Autodesk Inventor part; units mm, degrees
ref_plane "YZ Plane" through (0, 0, 0) normal (1, 0, 0) x (0, 1, 0)
ref_plane "XZ Plane" through (0, 0, 0) normal (0, 1, 0) x (-1, 0, 0)
ref_plane "XY Plane" through (0, 0, 0) normal (0, 0, 1) x (1, 0, 0)
sketch "Sketch1" plane through (0, 0, 0) normal (0, 0, 1) x (1, 0, 0)
  line L0 (0, 0) -> (125, 0)
  line L1 (125, 0) -> (125, 64)
  line L2 (125, 64) -> (0, 64)
  line L3 (0, 64) -> (0, 0)
  line L4 (0, 64) -> (14.15, 64) construction
  line L5 (14.15, 64) -> (14.15, 57.7) construction
  line L6 (14.15, 57.7) -> (110.85, 57.7)
  line L7 (110.85, 57.7) -> (110.85, 6.3)
  line L8 (110.85, 6.3) -> (14.15, 6.3)
  line L9 (14.15, 6.3) -> (14.15, 57.7)
  line L10 (0, 64) -> (0, 57.85) construction
  line L11 (0, 57.85) -> (6, 57.85) construction
  line L12 (6, 57.85) -> (6, 32.1) construction
  line L13 (6, 32.1) -> (6, 6.35) construction
  line L14 (6, 6.35) -> (119, 6.35) construction
  line L15 (119, 6.35) -> (119, 32.1) construction
  line L16 (119, 32.1) -> (119, 57.85) construction
  circle A0 centre (6, 57.85) radius 1.5
  circle A1 centre (6, 32.1) radius 1.5
  circle A2 centre (6, 6.35) radius 1.5
  circle A3 centre (119, 6.35) radius 1.5
  circle A4 centre (119, 57.85) radius 1.5
  circle A5 centre (119, 32.1) radius 1.5
  dimension "d0" = 125
  dimension "d1" = 64
  dimension "d2" = 14.15
  dimension "d3" = 6.3
  dimension "d4" = 96.7
  dimension "d5" = 51.4
  dimension "d6" = 6.15
  dimension "d7" = 6
  dimension "d8" = 25.75
  dimension "d9" = 25.75
  dimension "d10" = 113
  dimension "d11" = 3
  dimension "d12" = 3
  dimension "d13" = 3
  dimension "d14" = 3
  dimension "d16" = 3
  dimension "d18" = 3
extrude "Plate2" add sketch "Sketch1" along normal blind 0.5
sketch "Sketch2" plane through (0, 0, 0.5) normal (0, 0, 1) x (1, 0, 0)
  line L0 (0, 0) -> (125, 0)
  line L1 (125, 0) -> (125, -1)
  line L2 (125, -1) -> (0, -1)
  line L3 (0, -1) -> (0, 0)
  dimension "d20" = 125
  dimension "d21" = 1
sheet face with bend "Face3" sketch "Sketch2" thickness 0.5 toward (0, 0, -1) bend radius 0.5
bend "Bend1"
sketch "Sketch4" plane through (0, -1, 0.5) normal (0, -1, 0) x (1, 0, 0)
  line L0 (0, -0.5) -> (125, -0.5)
  line L1 (125, 0) -> (125, -0.5)
  line L2 (0, 0) -> (125, 0)
  line L3 (0, 0) -> (0, -0.5)
extrude "Extrusion1" add sketch "Sketch4" along normal blind 1.15
sketch "Sketch5" plane through (0, -1.65, 0.5) normal (0, -1, 0) x (1, 0, 0)
  line L0 (125, 0) -> (0, 0)
  line L1 (0, 0) -> (0, -140)
  line L2 (0, -140) -> (125, -140)
  line L3 (125, -140) -> (125, 0)
edge flange "Flange2" height 140 angle 90 thickness 0.5 bend radius 0.5 thickness toward (0, -1, 0) relief tear relief width 0.5 relief depth 0.25 edges at (62.5, -2.15, 0) wall of the first edge with corners at (125, -1.65, 0.5) (0, -1.65, 0.5) (0, -1.65, -139.5) (125, -1.65, -139.5)
bend "Bend3"
corner "Corner2"
sketch "Sketch6" plane through (0, -2.15, -139.5) normal (0, -1, 0) x (1, 0, 0)
  line L0 (0, 0) -> (0, 139)
  line L1 (125, 0) -> (0, 0)
  line L2 (125, 0) -> (120, 0) construction
  line L3 (120, 0) -> (120, 5) construction
  line L4 (120, 0) -> (110, 0) construction
  line L5 (110, 0) -> (110, 39.5) construction
  line L6 (110, 39.5) -> (15, 39.5) construction
  line L7 (15, 39.5) -> (110, 39.5)
  line L8 (110, 39.5) -> (110, 0)
  line L9 (110, 0) -> (15, 0)
  line L10 (15, 0) -> (15, 39.5)
  circle A0 centre (120, 5) radius 1.5
  line L11 (120, 5) -> (120, 15) construction
  line L12 (120, 15) -> (120, 25) construction
  circle A1 centre (120, 15) radius 1.5
  circle A2 centre (120, 25) radius 1.5
  line L13 (15, 0) -> (5, 0)
  circle A3 centre (5, 5) radius 1.5
  circle A4 centre (5, 15) radius 1.5
  circle A5 centre (5, 25) radius 1.5
  point P0 (0, 139.5)
  dimension "d49" = 5
  dimension "d50" = 5
  dimension "d51" = 10
  dimension "d52" = 39.5
  dimension "d53" = 95
  dimension "d54" = 3
  dimension "d55" = 10
  dimension "d56" = 10
  dimension "d57" = 3
  dimension "d58" = 3
  dimension "d59" = 10
  dimension "d60" = 3
  dimension "d61" = 3
  dimension "d62" = 3
extrude "Extrusion2" cut sketch "Sketch6" against normal blind 1.15
equation "\"d19\" = Thickness"
equation "\"d22\" = BendRadius"
equation "\"d23\" = BendReliefWidth"
equation "\"d25\" = MinimumRemnant"
equation "\"d24\" = BendReliefDepth"
equation "\"d26\" = TransitionRadius"
equation "\"d39\" = BendReliefWidth"
equation "\"d40\" = BendReliefDepth"
equation "\"d41\" = MinimumRemnant"
equation "\"d42\" = TransitionRadius"
equation "\"d45\" = BendRadius"
equation "\"d46\" = CornerReliefSize"
equation "\"d47\" = GapSize"
equation "\"d48\" = JacobiRadiusSize"
equation "\"BendRadius\" = Thickness"
equation "\"BendReliefWidth\" = Thickness"
equation "\"BendReliefDepth\" = 0.5 * Thickness"
equation "\"CornerReliefSize\" = 4 * Thickness"
equation "\"MinimumRemnant\" = 2 * Thickness"
equation "\"TransitionRadius\" = BendRadius"
equation "\"JacobiRadiusSize\" = BendRadius"
equation "\"GapSize\" = Thickness"
properties part number "psu mount"
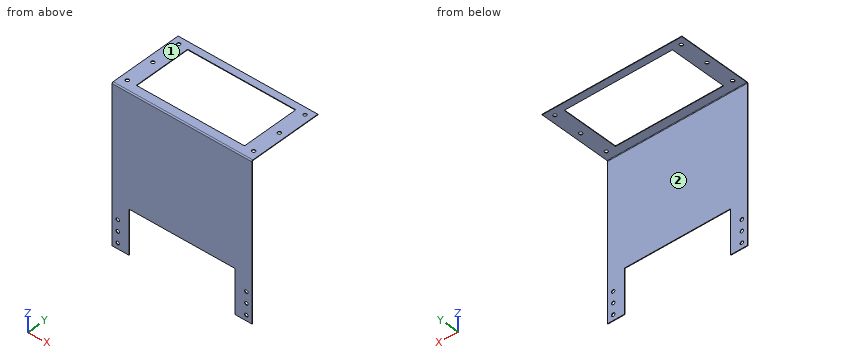
Build history of the part. All positions in model axes, mm. Face numbers are marked on the shaded views. A direction names the side the tool comes from. Give positions to 0.01 mm unless a question says otherwise; leave off trailing zeros. Order: outer loops, then holes, each group sorted by start corner. A loop starts at its lowest first (then second) coordinate and runs counter-clockwise, first axis right, second up. Notation, with made-up numbers: M 83.5,29 L 102.5,29 A23 ccw 102.5,42 Z; hole C 82,79.5 d10. An arc over 180 degrees is marked long. Return JSON: item names as keys, results as strings.
Q1. Wall check: probe 1 along X at (y, z) = (-1.8, -114.5); probe 2 along Y at (x, z) = (119, 0.35); probe 3 along Z at (x, y) = (120, -1.75). Give the ranges that are in metal, low to high. Write a range as from..to.
Answer list:
{"probe 1": "x = 0..3.5, 6.5..15, 110..118.5, 121.5..125", "probe 2": "y = -1.68..4.85, 7.85..30.6, 33.6..56.35, 59.35..64", "probe 3": "z = -139.5..-136, -133..-126, -123..-116, -113..0.3"}
Q2. Band-saw the part on B-B (x = 27.5). Give the cut face in (y, z).
Answer list:
{"outline": "M -2.15,-100 L -1.65,-100 L -1.65,-0.5 A0.5 cw -1.15,0 L 6.3,0 L 6.3,0.5 L -1.15,0.5 A1 ccw -2.15,-0.5 Z; M 57.7,0 L 64,0 L 64,0.5 L 57.7,0.5 Z"}
Q3. 3-axis set-ups, long thin cutter, end or side, ignore diameter. For the marked faces 1 and 2: which of +Z, -Z, +X, -X, +Y, -Y reach the whole face in a straight line?
Answer list:
{"face 1": "+Z, +X, -X, +Y, -Y", "face 2": "-Z, +X, -X, +Y"}
Q4. Band-saw the part on A-A (y = 39). Give the cut face in (x, z).
Answer list:
{"outline": "M 0,0 L 14.15,0 L 14.15,0.5 L 0,0.5 Z; M 110.85,0 L 125,0 L 125,0.5 L 110.85,0.5 Z"}
Q5. Band-saw the part on C-C (z = -83.5). Give the cut face in (x, y).
Answer list:
{"outline": "M 0,-2.15 L 125,-2.15 L 125,-1.65 L 0,-1.65 Z"}
Q6. Flat gauge pins, fed straight in: pin 1 (6 mm diameter, centred on x = 33.5, z = -25.5, fed in from +Y); pin 2 (4 mm diameter, centred on x = 6, y = 6.35, fed in from -Z). Where does each tip first touch, or does it go through?
Answer list:
{"pin 1": "stops at y = -1.65", "pin 2": "stops at z = 0"}
